from build123d import *

# Parameters (mm, degrees)
BOSS_EXTRUDE1_DEPTH  = 30
SHELL1_START         = 4
SHELL1_OUTLINE_W     = 57
SHELL1_OUTLINE_H     = 26
SHELL1_DEPTH         = 52
SKETCH2_W            = 9
SKETCH2_H            = 9
BOSS_EXTRUDE2_DEPTH  = 2
SKETCH3_W            = 9
SKETCH3_H            = 9
BOSS_EXTRUDE3_DEPTH  = 2
BOSS_EXTRUDE4_START  = -36.769553
SKETCH4_R            = 2.25
BOSS_EXTRUDE4_DEPTH  = 36.769553
M6_CLEARANCE_HOLE2_D = 6.6
M6_CLEARANCE_HOLE3_D = 6.6


# Read off the part's stored shape, not the designer's step: Shell1
with BuildPart() as part:
    # Sketch1 → Boss-Extrude1 (new body)
    with BuildSketch(Plane.XY):
        Polygon((0, 0), (60, 0), (0, 60), align=None)
    extrude(amount=-BOSS_EXTRUDE1_DEPTH)

    # Shell1 outline → Shell1 (cut)
    with BuildSketch(Plane.YZ.offset(SHELL1_START)):
        with Locations((32.5, -15)):
            Rectangle(SHELL1_OUTLINE_W, SHELL1_OUTLINE_H)
    extrude(amount=SHELL1_DEPTH, mode=Mode.SUBTRACT)

    # Sketch2 → Boss-Extrude2 (add)
    with BuildSketch(Plane(origin=(0, 4, 0), x_dir=(1, 0, 0), z_dir=(0, 1, 0))):
        with Locations((30, 15)):
            Rectangle(SKETCH2_W, SKETCH2_H)
    extrude(amount=BOSS_EXTRUDE2_DEPTH)

    # Sketch3 → Boss-Extrude3 (add)
    with BuildSketch(Plane(origin=(4, 0, 0), x_dir=(0, 0, -1), z_dir=(1, 0, 0))):
        with Locations((15, 43.5)):
            Rectangle(SKETCH3_W, SKETCH3_H)
    extrude(amount=BOSS_EXTRUDE3_DEPTH)

    # Sketch4 → Boss-Extrude4 (add)
    # profile 1 of 2: a face of its own
    with BuildSketch(Plane(origin=(30, 30, 0), x_dir=(0, 0, -1), z_dir=(0.7071067811865477, 0.7071067811865475, 0)).offset(BOSS_EXTRUDE4_START)):
        with BuildLine():
            Line((2, 3), (2, -3))
            Line((2, -3), (5, -3))
            ThreePointArc((5, -3), (8, 0), (5, 3))
            Line((5, 3), (2, 3))
        make_face()
        with Locations(Location((5, 0, 0), (0, 0, 90))):
            Circle(SKETCH4_R, mode=Mode.SUBTRACT)
    # profile 2 of 2: a face of its own
    with BuildSketch(Plane(origin=(30, 30, 0), x_dir=(0, 0, -1), z_dir=(0.7071067811865477, 0.7071067811865475, 0)).offset(BOSS_EXTRUDE4_START)):
        with BuildLine():
            Line((25, -3), (28, -3))
            Line((28, -3), (28, 3))
            Line((28, 3), (25, 3))
            ThreePointArc((25, 3), (22, 0), (25, -3))
        make_face()
        with Locations(Location((25, 0, 0), (0, 0, 90))):
            Circle(SKETCH4_R, mode=Mode.SUBTRACT)
    extrude(amount=BOSS_EXTRUDE4_DEPTH)

    # M6 Clearance Hole2 (through all)
    with Locations(Plane(origin=(0, 6, 0), x_dir=(1, 0, 0), z_dir=(0, 1, 0))):
        with Locations((30, 15)):
            Hole(M6_CLEARANCE_HOLE2_D / 2)

    # M6 Clearance Hole3 (through all)
    with Locations(Plane(origin=(6, 0, 0), x_dir=(0, 0, -1), z_dir=(1, 0, 0))):
        with Locations((15, 43.5)):
            Hole(M6_CLEARANCE_HOLE3_D / 2)


solid = part.part
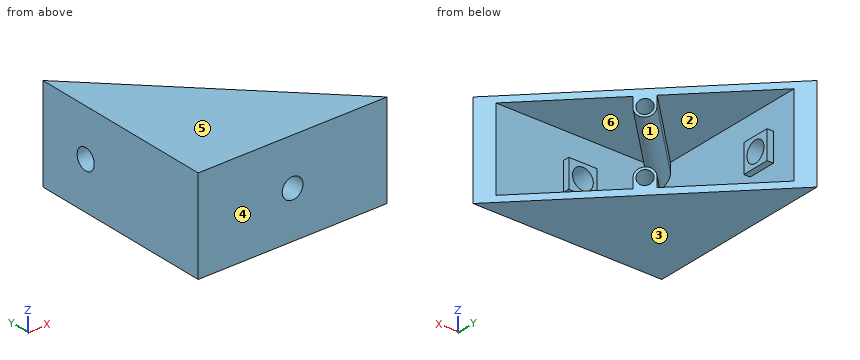
Check sheet for the modelled part. Datum: model origin and axes. Units: mm. Face numbers are marked on the shaded views. A direction names the side the tool comes from. Give positions to 0.01 mm unless a question says otherwise; leave off trailing zeros. Loops run counter-clockwise (first coordinate to the right, second up) from the corner with the lowest first, then second, coordinate; pieces in that order, holes last. Notation, with made-up numbers: M 78.5,24 L 95.5,24 A20 cw 95.5,63 Z; hole C 80.5,-32 d9. An arc over 180 degrees is marked long. Return JSON: item names as keys, results as strings. Group by question number.
1. Cross-section at D-D on y = 50. Record the boundary of the cut face in (x, z).
2. Cross-section at B-B on x = 46. Record the boundary of the cut face in (y, z).
3. Go/stop test with flat-tipped pins: pin 1 (1.6 mm diameter, centred on y = 6, z = -24, fed in from +X); pin 2 (2.5 mm diameter, centred on y = 5.5, z = -5, fed in from +X); pin 3 (13 mm diameter, centred on y = 29, z = -20.5, fed in from +X). Record where each tip stops, or that it passes through.
4. Cross-section at A-A on z = -15. Record the boundary of the cut face in (x, y).
5. Tool access check on the marked faces 1, 2 and 3. Record the directions out of +Z, -Z, +X, -X, +Y, -Y that give a thin tool (end or side, any length) a straight path to the whole face; none if there is none.
6. Cross-section at C-C on y = 43.5. Record the boundary of the cut face in (x, z), plus the area to 3 significant figures.
7. Mould release check, pull along Z, two halves, no side actions. Record for the marked faces 4, 5 and 6: released by +Z, released by -Z, zero draft, split by the parting line, or undercut.
8. Thickness scan on L1, parallel to X at y = 4.1, z = -15; L2, parallel to Z at x = 40, y = 14.5; L3, parallel to Z at x = 23.5, y = 26. Record the ranges inside material, lowest first.
Return value:
{
 "1": {"outline": "M 0,-30 L 10,-30 L 10,-28 L 4,-28 L 4,-2 L 10,-2 L 10,0 L 0,0 Z"},
 "2": {"outline": "M 0,-30 L 14,-30 L 14,-28 L 4,-28 L 4,-2 L 14,-2 L 14,0 L 0,0 Z"},
 "3": {"pin 1": "x = 10.87", "pin 2": "x = 10.99", "pin 3": "x = 32.12"},
 "4": {"outline": "M 0,0 L 26.7,0 L 26.7,6 L 25.5,6 L 25.5,4 L 4,4 L 4,39 L 6,39 L 6,40.2 L 0,40.2 Z; M 0,46.8 L 6,46.8 L 6,48 L 4,48 L 4,56 L 0,60 Z; M 33.3,0 L 60,0 L 56,4 L 34.5,4 L 34.5,6 L 33.3,6 Z"},
 "5": {"face 1": "none", "face 2": "+Y", "face 3": "-Z, +X, -X, +Y, -Y"},
 "6": {"outline": "M 0,-30 L 16.5,-30 L 16.5,-28 L 4,-28 L 4,-19.5 L 6,-19.5 L 6,-18.3 L 0,-18.3 Z; M 0,-11.7 L 6,-11.7 L 6,-10.5 L 4,-10.5 L 4,-2 L 16.5,-2 L 16.5,0 L 0,0 Z", "area": "148 mm^2"},
 "7": {"face 4": "zero draft", "face 5": "released by +Z", "face 6": "undercut"},
 "8": {"L1": "0 to 4, 25.5 to 26.7, 33.3 to 34.5", "L2": "-30 to -28, -2 to 0", "L3": "-30 to -26.39, -23.61 to -22.58, -7.42 to -6.39, -3.61 to 0"}
}
